Part print with two shaded views. Sizes in mm from the minimum x, y, z corner. A direction names the side the tool comes from. Coordinates: 2 decimals unless noted, no trailing zeros. Loops run counter-clockwise (first coordinate to the right, second up) from the corner with the lowest first, then second, coordinate; pieces in that order, holes last.
Item 1: Cut at A-A (z = 8.5). List the corners of the cut face in (x, y).
Item 2: Cut at C-C (x = 23.5). List the corners of the cut face in (y, z).
Item 3: Mould opens along X. For the marked faces 4, 5 and 6 say: released by +X, released by -X, zero draft, split by the parting line, or undercut.
Item 4: Drill centre lines: line 1 along X through (y, z) = (23.5, 2.75); line 2 along Z through (x, y) = (13.5, 2.5); line 3 along Z through (x, y) = (25, 25). Where is each one in solid material? Low to high.
Item 5: Cut at D-D (y = 24.5). List the corners of the cut face in (x, z).
Item 6: Flat gauge pins, fed straight in: pin 1 (8.5 mm diameter, centred on x = 14.5, y = 9.5, fed in from +Z); pin 2 (10 mm diameter, centred on x = 29, y = 22.5, fed in from +Z); pin 3 (5 mm diameter, centred on x = 43, z = 5, fed in from +Y); pin 4 (2 mm diameter, centred on x = 22, y = 9, fed in from +Z). Where does each tip first touch, or does it go through?
Item 7: 3-axis set-ups, long thin cutter, end or side, ignore diameter. For the marked faces 1, 2 and 3: which of +Z, -Z, +X, -X, +Y, -Y reach the whole face in a straight line?
Item 8: Cut at B-B (y = 14.25). List the corners of the cut face in (x, z).
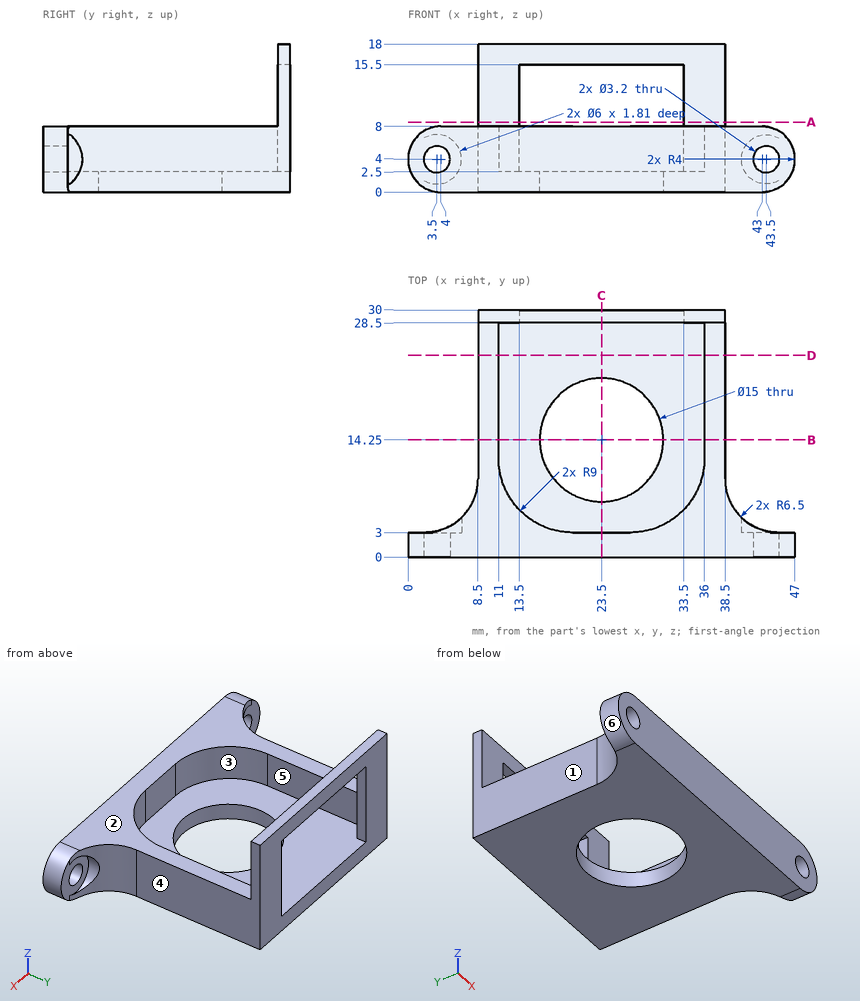
Filled sheet:
1. outline: (8.5, 28.5) - (13.5, 28.5) - (13.5, 30) - (8.5, 30) - close; (33.5, 28.5) - (38.5, 28.5) - (38.5, 30) - (33.5, 30) - close
2. outline: (0, 0) - (6.75, 0) - (6.75, 2.5) - (3, 2.5) - (3, 8) - (0, 8) - close; (21.75, 0) - (30, 0) - (30, 2.5) - (21.75, 2.5) - close; (28.5, 15.5) - (30, 15.5) - (30, 18) - (28.5, 18) - close
3. face 4: released by +X
3. face 5: undercut
3. face 6: released by -X
4. line 1: x = 8.5 to 11, 36 to 38.5
4. line 2: z = 0 to 8
4. line 3: z = 0 to 2.5
5. outline: (8.5, 0) - (38.5, 0) - (38.5, 8) - (36, 8) - (36, 2.5) - (11, 2.5) - (11, 8) - (8.5, 8) - close
6. pin 1: stops at z = 8
6. pin 2: stops at z = 2.5
6. pin 3: stops at y = 4.81
6. pin 4: passes through
7. face 1: +Z, -Z, -X, +Y
7. face 2: +Z, +X, -X, -Y
7. face 3: +Z
8. outline: (8.5, 0) - (16, 0) - (16, 2.5) - (11, 2.5) - (11, 8) - (8.5, 8) - close; (31, 0) - (38.5, 0) - (38.5, 8) - (36, 8) - (36, 2.5) - (31, 2.5) - close
